Can you work these out from the model? Positions are in its coordinate system, mm. A direction names the side the tool comes from. Coordinates: 2 decimals unless noted, no trailing zeros. Order: outer loops, then holes, each group sorted by start corner. A loop starts at its lowest first (then second) coordinate and runs counter-clockwise, first axis right, second up. Notation, with made-up numbers: (-30.75, 41.25) - (-18.75, 41.25) arc R19 cw to (-18.75, 51.25) - close; hole circle Ø11 at (60.5, 9). An arc over 180 degrees is marked (long way). Return JSON: item names as keys, results as strings. Group by question number.
1) For pin 1 Ø1 at (y, z) = (-40.5, 1) entering from +X; pin 2 Ø1.5 at (y, z) = (-33, 1.5) entering from -X; pin 3 Ø1.6 at (x, z) = (80.5, 2) entering from -Y, each with a flat end and sliding along its axis, tell me the tip position at first contact or that it passes through.
2) Which directions (+Z, -Z, +X, -X, +Y, -Y) give clear straight access to the entire face, cutting with the end or side of a thin tool? Please do faces 1 (the face through (-32, -24.073, 2)), 2 (the face through (40, 38.898, 2)), 3 (the face through (-79.5, 26, 2)), 4 (the face through (-79.5, -26, 2)), 5 (the face through (-10, -41, 2)).
3) Imagine slicing it at A-A (x = 27). Write out the boundary of the cut face in (y, z) (3 decimals).
4) If I drill on line 1 along X through (y, z) = (-21, 1.8); line 2 along Y through (x, z) = (47.5, 1.15); line 3 along Y through (x, z) = (-27, 1.2), over which ranges is the centre line in solid material (lowest first)?
5) Imagine slicing it at D-D (x = -0.5). Write out the boundary of the cut face in (y, z) (3 decimals), and give its area (3 significant figures).
6) If we mould it in two halves opening along Y, with no side actions, what happens to faces 6 (the face through (-40, 38.898, 2)), 7 (the face through (-21.5, -18, 2)), 8 (the face through (-30, -41, 2))? For each: pulls with the +Y half, pulls with the -Y half, needs draft (parallel to the pull), parting line crosses it, or undercut.
7) Imagine slicing it at C-C (z = 0.9). Give the number of separate pieces and of enclosed holes in the cut face, and give its area (3 significant figures).
8) Imagine slicing it at B-B (y = 14). Write out the boundary of the cut face in (x, z) (3 decimals), and give its area (3 significant figures).
```python
from build123d import *

# Parameters (mm, degrees)
ESQUISSE1_W             = 165.35
ESQUISSE1_H             = 84.146
BOSS_EXTRU_1_DEPTH      = 3.175
ESQUISSE2_W             = 3.175
ESQUISSE2_H             = 32.073
ENL_V_MAT_EXTRU_1_DEPTH = 93.819036727
ESQUISSE3_W             = 20
ESQUISSE3_H             = 3.175
ENL_V_MAT_EXTRU_2_DEPTH = 93.819036727
ESQUISSE5_W             = 22
ESQUISSE5_H             = 12
ENL_V_MAT_EXTRU_3_DEPTH = 93.819036727
CONG_1_R                = 3
CONG_1_OF_SYM_TRIE3_R   = 3


with BuildPart() as part:
    # Esquisse1 → Boss.-Extru.1 (new body)
    with BuildSketch(Plane.XY):
        Rectangle(ESQUISSE1_W, ESQUISSE1_H)
    extrude(amount=BOSS_EXTRU_1_DEPTH)

    # Esquisse2 → Enlèv. mat.-Extru.1 (cut, through all)
    with BuildSketch(Plane.XY.offset(3.175)):
        with Locations((-81.0875, -26.0365)):
            Rectangle(ESQUISSE2_W, ESQUISSE2_H)
        with Locations((-81.0875, 26.0365)):
            Rectangle(ESQUISSE2_W, ESQUISSE2_H)
    enl_v_mat_extru_1 = extrude(amount=-ENL_V_MAT_EXTRU_1_DEPTH, mode=Mode.SUBTRACT)

    # Symétrie1: Enlèv. mat.-Extru.1 across plane
    add(enl_v_mat_extru_1.mirror(Plane(origin=(0, 0, 0), x_dir=(0, 0, 1), z_dir=(1, 0, 0))), mode=Mode.SUBTRACT)

    # Esquisse3 → Enlèv. mat.-Extru.2 (cut, through all)
    with BuildSketch(Plane.XY.offset(3.175)):
        with Locations((0, -40.4855)):
            Rectangle(ESQUISSE3_W, ESQUISSE3_H)
        with Locations((40, -40.4855)):
            Rectangle(ESQUISSE3_W, ESQUISSE3_H)
        with Locations((-40, -40.4855)):
            Rectangle(ESQUISSE3_W, ESQUISSE3_H)
    enl_v_mat_extru_2 = extrude(amount=-ENL_V_MAT_EXTRU_2_DEPTH, mode=Mode.SUBTRACT)

    # Symétrie2: Enlèv. mat.-Extru.2 across plane
    add(enl_v_mat_extru_2.mirror(Plane.ZX), mode=Mode.SUBTRACT)

    # Esquisse5 → Enlèv. mat.-Extru.3 (cut, through all)
    with BuildSketch(Plane.XY.offset(3.175)):
        with Locations((32.5, -18.073)):
            Rectangle(ESQUISSE5_W, ESQUISSE5_H)
    enl_v_mat_extru_3 = extrude(amount=-ENL_V_MAT_EXTRU_3_DEPTH, mode=Mode.SUBTRACT)

    # Congé1
    cong_1_edges = [part.edges().sort_by_distance(p)[0] for p in [
        (21.5, -24.073, 1.5875),
        (21.5, -12.073, 1.5875),
        (43.5, -12.073, 1.5875),
        (43.5, -24.073, 1.5875),
    ]]
    fillet(cong_1_edges, radius=CONG_1_R)

    # Symétrie3: Enlèv. mat.-Extru.3 across plane
    add(enl_v_mat_extru_3.mirror(Plane(origin=(0, 0, 0), x_dir=(0, 0, 1), z_dir=(1, 0, 0))), mode=Mode.SUBTRACT)

    # Congé1 of Symétrie3
    cong_1_of_sym_trie3_edges = [part.edges().sort_by_distance(p)[0] for p in [
        (-21.5, -24.073, 1.5875),
        (-21.5, -12.073, 1.5875),
        (-43.5, -12.073, 1.5875),
        (-43.5, -24.073, 1.5875),
    ]]
    fillet(cong_1_of_sym_trie3_edges, radius=CONG_1_OF_SYM_TRIE3_R)


solid = part.part
```
Calculated:
{
 "1": {"pin 1": "x = 79.5", "pin 2": "x = -79.5", "pin 3": "y = -10"},
 "2": {"face 1": "+Z, -Z", "face 2": "+Z, -Z, +Y", "face 3": "+Z, -Z, -X, +Y", "face 4": "+Z, -Z, -X, -Y", "face 5": "+Z, -Z, -Y"},
 "3": {"outline": "(-42.073, 0) - (-24.073, 0) - (-24.073, 3.175) - (-42.073, 3.175) - close; (-12.073, 0) - (42.073, 0) - (42.073, 3.175) - (-12.073, 3.175) - close"},
 "4": {"line 1": "-79.5 to -43.5, -21.5 to 21.5, 43.5 to 79.5", "line 2": "-38.9 to 38.9", "line 3": "-42.07 to -24.07, -12.07 to 42.07"},
 "5": {"outline": "(-38.898, 0) - (38.898, 0) - (38.898, 3.175) - (-38.898, 3.175) - close", "area": "247 mm2"},
 "6": {"face 6": "pulls with the +Y half", "face 7": "undercut", "face 8": "needs draft"},
 "7": {"separate pieces": "1", "enclosed holes": "2", "area": "12,600 mm2"},
 "8": {"outline": "(-79.5, 0) - (79.5, 0) - (79.5, 3.175) - (-79.5, 3.175) - close", "area": "505 mm2"}
}
